Geometry check sheet. Reference: the model listing, model coordinates, mm. A direction names the side the tool comes from. Coordinates: 2 decimals unless noted, no trailing zeros. Loops run counter-clockwise (first coordinate to the right, second up) from the corner with the lowest first, then second, coordinate; pieces in that order, holes last. Notation, with made-up numbers: (-13.5, 74.5) -> (-1.5, 74.5) arc R17 cw to (-1.5, 98.5) -> close; hole circle Ø8 at (68, -38). An arc over 180 degrees is marked (long way). Answer as a JSON object with one key per item and string values.
from build123d import *

# Parameters (mm, degrees)
SKETCH1_W           = 673.1
SKETCH1_H           = 120.7008
BOSS_EXTRUDE1_DEPTH = 19.05
SKETCH3_W           = 30.013638179
SKETCH3_H           = 33.61527476
CUT_EXTRUDE5_DEPTH  = 20.05
SKETCH2_R           = 12.7
CUT_EXTRUDE4_DEPTH  = 20.05
SKETCH4_W           = 19.05
SKETCH4_H           = 19.05
CUT_EXTRUDE6_DEPTH  = 20.05


with BuildPart() as part:
    # Sketch1 → Boss-Extrude1 (new body)
    with BuildSketch(Plane(origin=(0, 0, 0), x_dir=(1, 0, 0), z_dir=(0, 1, 0))):
        with Locations((336.55, 60.3504)):
            Rectangle(SKETCH1_W, SKETCH1_H)
    extrude(amount=BOSS_EXTRUDE1_DEPTH)

    # Sketch3 → Cut-Extrude5 (cut, through all)
    with BuildSketch(Plane.XZ):
        with Locations((590.529823595, -44.616403279)):
            Rectangle(SKETCH3_W, SKETCH3_H)
    extrude(amount=-CUT_EXTRUDE5_DEPTH, mode=Mode.SUBTRACT)

    # Sketch2 → Cut-Extrude4 (cut, through all)
    with BuildSketch(Plane.XZ):
        with Locations((341.9094, -105.5624)):
            Circle(SKETCH2_R)
    extrude(amount=-CUT_EXTRUDE4_DEPTH, mode=Mode.SUBTRACT)

    # Sketch4 → Cut-Extrude6 (cut, through all)
    with BuildSketch(Plane.XZ):
        with Locations((663.575, -9.525)):
            Rectangle(SKETCH4_W, SKETCH4_H)
        with Locations((9.525, -111.1758)):
            Rectangle(SKETCH4_W, SKETCH4_H)
    extrude(amount=-CUT_EXTRUDE6_DEPTH, mode=Mode.SUBTRACT)


solid = part.part
1. Section check B-B, the plane z = -52. Record the boundary of the cut face in (x, y).
Evaluation:
{"outline": "(0, 0) -> (575.52, 0) -> (575.52, 19.05) -> (0, 19.05) -> close; (605.54, 0) -> (673.1, 0) -> (673.1, 19.05) -> (605.54, 19.05) -> close"}
2. Depth check by flat-ended pin: P1, Ø9.5, axis at y = 7, z = -8, coming from the +X side; P2, Ø8, axis at y = 9.5, z = -25.5, coming from the -X side; P3, Ø9.5, axis at x = 664, y = 13, coming from the +Z side. Enter the tip coordinate at first touch or a pass-through.
Evaluation:
{"P1": "stops at x = 654.05", "P2": "stops at x = 0", "P3": "stops at z = -19.05"}
3. Section check A-A, the plane x = 598.5. Record the boundary of the cut face in (y, z).
Evaluation:
{"outline": "(0, -120.7) -> (19.05, -120.7) -> (19.05, -61.42) -> (0, -61.42) -> close; (0, -27.81) -> (19.05, -27.81) -> (19.05, 0) -> (0, 0) -> close"}
4. Section check D-D, the plane z = -10. Record the boundary of the cut face in (x, y).
Evaluation:
{"outline": "(0, 0) -> (654.05, 0) -> (654.05, 19.05) -> (0, 19.05) -> close"}
5. Section check C-C, the plane y = 7.5. Record the boundary of the cut face in (x, z).
Evaluation:
{"outline": "(0, -101.65) -> (19.05, -101.65) -> (19.05, -120.7) -> (673.1, -120.7) -> (673.1, -19.05) -> (654.05, -19.05) -> (654.05, 0) -> (0, 0) -> close; hole circle Ø25.4 at (341.91, -105.56); hole (575.52, -61.42) -> (605.54, -61.42) -> (605.54, -27.81) -> (575.52, -27.81) -> close"}
6. Mould release check, pull along X, two halves, no side actions. Record for faces 1 (the face through (575.523, 9, -45)), 2 (the face through (590, 9, -27.809)), 3 (the face through (673.1, 9, -69)), 4 (the face through (332, 0, -61)): released by +X, released by -X, zero draft, split by the parting line, or undercut.
Evaluation:
{"face 1": "undercut", "face 2": "undercut", "face 3": "released by +X", "face 4": "zero draft"}
7. Tool access check on faces 5 (the face through (605.537, 9, -45)), 6 (the face through (9, 9, -101.651)), 7 (the face through (663, 9, -19.05)). Record the directions out of +Z, -Z, +X, -X, +Y, -Y that give a thin tool (end or side, any length) a straight path to the whole face; none if there is none.
Evaluation:
{"face 5": "+Y, -Y", "face 6": "-Z, -X, +Y, -Y", "face 7": "+Z, +X, +Y, -Y"}
8. Thickness scan on probe 1 along X at (y, z) = (8.75, -36); probe 2 along Z at (x, y) = (577.5, 7.5); probe 3 along X at (y, z) = (16.75, -99). Record the ranges inside material, lowest first. Write a range as from..to.
Evaluation:
{"probe 1": "x = 0..575.52, 605.54..673.1", "probe 2": "z = -120.7..-61.42, -27.81..0", "probe 3": "x = 0..331.04, 352.78..673.1"}
